```python
from build123d import *

# Parameters (mm, degrees)
CROQUIS1_W              = 15
CROQUIS1_H              = 20
CROQUIS1_R              = 1.5
SALIENTE_EXTRUIR1_DEPTH = 3
CROQUIS2_R              = 1
CORTAR_EXTRUIR1_DEPTH   = 10


with BuildPart() as part:
    # Croquis1 → Saliente-Extruir1 (new body)
    with BuildSketch(Plane(origin=(0, 0, 0), x_dir=(0, 0, -1), z_dir=(1, 0, 0))):
        with Locations((-10.5, 0)):
            Rectangle(CROQUIS1_W, CROQUIS1_H)
        Polygon((0, 0), (0, -10), (18, -10), (18, 10), (0, 10), align=None)
        with Locations((6, 0)):
            Circle(CROQUIS1_R, mode=Mode.SUBTRACT)
        with Locations((13, 0)):
            Circle(CROQUIS1_R, mode=Mode.SUBTRACT)
        Polygon((-3, 10), (-3, -10), (0, -10), (0, 0), (0, 10), align=None)
    extrude(amount=SALIENTE_EXTRUIR1_DEPTH)

    # Croquis2 → Cortar-Extruir1 (cut)
    with BuildSketch(Plane(origin=(3, 0, 0), x_dir=(0, 0, -1), z_dir=(1, 0, 0))):
        with Locations((-14, 6)):
            Circle(CROQUIS2_R)
        with Locations((-6, -6)):
            Circle(CROQUIS2_R)
    extrude(amount=-CORTAR_EXTRUIR1_DEPTH, mode=Mode.SUBTRACT)


solid = part.part
```
Work out the finished part from the listing and answer in its coordinate system (mm). Round coordinates to 2 decimals unless told otherwise and drop trailing zeros. Order: outer loops, then holes, each group sorted by start corner. A loop starts at its lowest first (then second) coordinate and runs counter-clockwise, first axis right, second up.
Q1. A cutting plane is placed at B-B, the plane z = 14. Determine the outline of the cut face in (x, y), then the cut area to 3 significant figures.
Solution:
outline: (0, -10) - (3, -10) - (3, 5) - (0, 5) - close; (0, 7) - (3, 7) - (3, 10) - (0, 10) - close
area: 54.0 mm2
Q2. Find the intervals of material crossed by line 1 along Z through (x, y) = (1.95, -0.5); line 2 along Y through (x, z) = (1.2, 14); line 3 along Y through (x, z) = (0.85, -13), in increasing order.
Solution:
line 1: z = -18 to -14.41, -11.59 to -7.41, -4.59 to 18
line 2: y = -10 to 5, 7 to 10
line 3: y = -10 to -1.5, 1.5 to 10
Q3. A cutting plane is placed at D-D, the plane y = 0. Determine the outline of the cut face in (x, z), then the cut area to 3 significant figures.
Solution:
outline: (0, -18) - (3, -18) - (3, -14.5) - (0, -14.5) - close; (0, -11.5) - (3, -11.5) - (3, -7.5) - (0, -7.5) - close; (0, -4.5) - (3, -4.5) - (3, 18) - (0, 18) - close
area: 90.0 mm2
Q4. A cutting plane is placed at A-A, the plane y = 6. Determine the outline of the cut face in (x, z), then the cut area to 3 significant figures.
Solution:
outline: (0, -18) - (3, -18) - (3, 13) - (0, 13) - close; (0, 15) - (3, 15) - (3, 18) - (0, 18) - close
area: 102 mm2
Q5. A cutting plane is placed at C-C, the plane x = 2.1. Determine the outline of the cut face in (y, z).
Solution:
outline: (-10, -18) - (10, -18) - (10, 18) - (-10, 18) - close; hole circle Ø2 at (-6, 6); hole circle Ø3 at (0, -13); hole circle Ø3 at (0, -6); hole circle Ø2 at (6, 14)
Q6. The mould has two halves that part along Y. Classify faces 1 (the flat face through (1, -10, 0)), 2 (the cylindrical face through (1.521, -5.324, 6.737)), 3 (the flat face through (1, 0, -18)), 4 (the cylindrical face through (1.48, 0.07, -11.5)): pulls with the +Y half, pulls with the -Y half, needs draft (parallel to the pull), parting line crosses it, or undercut.
Solution:
face 1: pulls with the -Y half
face 2: undercut
face 3: needs draft
face 4: undercut
